Can you work these out from the drawing? Everything is in mm from the part's minimum corner. Round coordinates to 2 decimals unless told otherwise and drop trailing zeros. Write each loop counter-clockwise with the first axis right and the second up, starting at its lowest first coordinate (ties: lowest second). Pieces come first, ordered by that corner, then holes. Notation, with made-up numbers: (-4, 83.5) - (27, 83.5) arc R21 ccw to (27, 101.5) - close; hole circle Ø2 at (-16.5, -33). An arc over 180 degrees is marked (long way). One line per item, written item: value. Start each with the question number.
(1) If I drill on L1, parallel to Y at x = 1.55, z = 3 (3 decimals); L2, parallel to Y at x = 2.7, z = 5 (3 decimals); L3, parallel to Z at x = 2.55, y = 74 (3 decimals), over which ranges is the centre line in solid material (lowest first)? Write a range as from..to.
(2) I want a section at B-B on y = 72.5. List the corners of the cut face in (x, z) for me (3 decimals), plus the area to 3 significant figures.
(3) I want a section at C-C on z = 32.5. List the corners of the cut face in (x, y) for me (3 decimals), plus the area to 3 significant figures.
(4) I want a section at A-A on x = 1.95. List the corners of the cut face in (y, z) for me (3 decimals), plus the area to 3 significant figures.
(5) I'm going to push flat-ended pins straight in: pin 1 Ø1 at (x, z) = (2, 8) entering from +Y (3 decimals); pin 2 Ø1.6 at (x, y) = (2, 71) entering from -Z (3 decimals). Where does each tip first touch, or does it pass through?
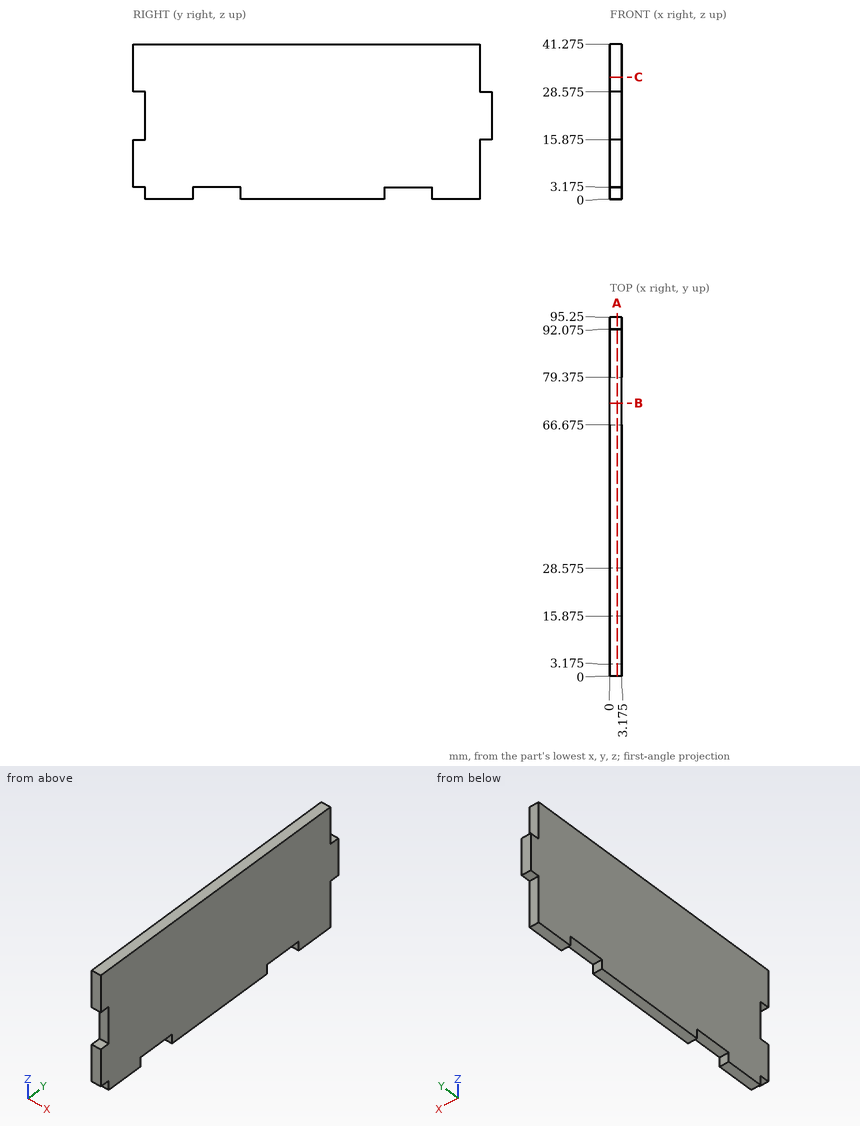
Established:
1. L1: 3.175..15.875, 28.575..66.675, 79.375..92.075
1. L2: 0..92.075
1. L3: 3.175..41.275
2. outline: (0, 3.175) - (3.175, 3.175) - (3.175, 41.275) - (0, 41.275) - close
2. area: 121 mm2
3. outline: (0, 0) - (3.175, 0) - (3.175, 92.075) - (0, 92.075) - close
3. area: 292 mm2
4. outline: (0, 3.175) - (3.175, 3.175) - (3.175, 0) - (15.875, 0) - (15.875, 3.175) - (28.575, 3.175) - (28.575, 0) - (66.675, 0) - (66.675, 3.175) - (79.375, 3.175) - (79.375, 0) - (92.075, 0) - (92.075, 15.875) - (95.25, 15.875) - (95.25, 28.575) - (92.075, 28.575) - (92.075, 41.275) - (0, 41.275) - (0, 28.575) - (3.175, 28.575) - (3.175, 15.875) - (0, 15.875) - close
4. area: 3,710 mm2
5. pin 1: y = 92.075
5. pin 2: z = 3.175
